Input: part model. Units: mm. Frame: model coordinates. A direction names the side the tool comes from. Round coordinates to 2 decimals unless told otherwise and drop trailing zeros. Loops run counter-clockwise (first coordinate to the right, second up) from the corner with the lowest first, then second, coordinate; pieces in that order, holes last.
1) Draft query along X for faces 1 (the face through (-53, 1, 35.19)), 2 (the face through (46.445, 1.479, 54.256)), 3 (the face through (42, 1, 38.19)). Return one class per face: pulls with the +X half, pulls with the -X half, needs draft (parallel to the pull), parting line crosses it, or undercut.
2) Ray query, line 1 along X through (y, z) = (0.4, 41); line 2 along X through (y, z) = (2.6, 54); line 3 along X through (y, z) = (1.25, 37.5). Return the intervals inside material, ascending.
3) Section A-A, the plane z = 45.5. Return loops of the section in (x, y).
4) Section D-D, the plane x = 26. Return loops of the section in (y, z).
5) First-contact query: pin 1 (0.9 mm diameter, centred on x = -47, y = 2, fed in from -Z); pin 2 (1.5 mm diameter, centred on x = 3.5, y = 2, fed in from -Z); pin 3 (0.9 mm diameter, centred on y = 1.5, z = 41.5, fed in from +X); pin 4 (0.9 mm diameter, centred on y = 1.5, z = 47, fed in from +X). Flat tips, straight axial feed; report the tip coordinate or a pass-through.
6) Section B-B, the plane y = 1.2. State how many separate pieces and enclosed holes the cut face has, and give its area (3 significant figures).
7) Access query for faces 4 (the face through (-55.419, 1, 41)), 5 (the face through (18.229, 1.521, 62.266)), 6 (the face through (31.581, 1, 58)). Directions: +Z, -Z, +X, -X, +Y, -Y. A direction counts if a zero-diameter tool reaches every point of the face in a straight line with its end or side. Return the directions, or none.
8) Section C-C, the plane x = 6. Return loops of the section in (y, z).
from build123d import *

# Parameters (mm, degrees)
BOSS_EXTRUDE1_DEPTH = 3
FILLET2_R           = 2.5
FILLET3_R           = 1
FILLET5_R           = 2.5
FILLET6_R           = 5
FILLET7_R           = 25


with BuildPart() as part:
    # Sketch1 → Boss-Extrude1 (new body)
    with BuildSketch(Plane(origin=(0, 0, 0), x_dir=(1, 0, 0), z_dir=(0, 1, 0))):
        with BuildLine():
            Line((-62.418566214, -47.190177149), (-58.418566214, -47.190177149))
            Line((-58.418566214, -47.190177149), (-58.418566214, -35.190177149))
            Line((-58.418566214, -35.190177149), (-48.418566214, -35.190177149))
            Line((-48.418566214, -35.190177149), (-48.418566214, -47.190177149))
            Line((-48.418566214, -47.190177149), (-44.418566214, -47.190177149))
            Line((-44.418566214, -47.190177149), (-43.418817081, -57.187668474))
            Line((-43.418817081, -57.187668474), (-43.418817081, -59.137504987))
            Line((-43.418817081, -59.137504987), (-40.418817081, -59.137504987))
            Line((-40.418817081, -59.137504987), (-40.418817081, -57.137504987))
            Line((-40.418817081, -57.137504987), (-38.722684913, -52.023499684))
            ThreePointArc((-38.722684913, -52.023499684), (-37.561438496, -51.091888176), (-36.235977812, -51.769787298))
            Line((-36.235977812, -51.769787298), (-33.13692456, -57.137504987))
            Line((-33.13692456, -57.137504987), (28.581433786, -57.137504987))
            Line((28.581433786, -57.137504987), (28.581433786, -59.137504987))
            Line((28.581433786, -59.137504987), (31.581433786, -59.137504987))
            Line((31.581433786, -59.137504987), (31.581433786, -57.187643384))
            Line((31.581433786, -57.187643384), (32.581433786, -47.190177149))
            Line((32.581433786, -47.190177149), (36.581433786, -47.190177149))
            Line((36.581433786, -47.190177149), (36.581433786, -35.190177149))
            Line((36.581433786, -35.190177149), (46.581433786, -35.190177149))
            Line((46.581433786, -35.190177149), (46.581433786, -47.190177149))
            Line((46.581433786, -47.190177149), (50.581433786, -47.190177149))
            Line((50.581433786, -47.190177149), (41.830568429, -62.137504987))
            ThreePointArc((41.830568429, -62.137504987), (30.081433786, -65.137504987), (18.332299143, -62.137504987))
            Line((18.332299143, -62.137504987), (-26.340663857, -62.360316421))
            ThreePointArc((-26.340663857, -62.360316421), (-40.074739293, -66.344446247), (-53.758312176, -62.190177149))
            Line((-53.758312176, -62.190177149), (-62.202371167, -57.642224353))
            ThreePointArc((-62.202371167, -57.642224353), (-62.450096964, -57.079754395), (-61.965274707, -56.702013871))
            Line((-61.965274707, -56.702013871), (-59.524980934, -56.702013871))
            ThreePointArc((-59.524980934, -56.702013871), (-58.225942828, -55.952013871), (-58.225942828, -54.452013871))
            Line((-58.225942828, -54.452013871), (-62.418566214, -47.190177149))
        make_face()
        Polygon((36.547763078, -51.190177149), (39.581433786, -51.190177149), (39.581433786, -44.190177149), (39.581433786, -38.190177149), (43.581433786, -38.190177149), (43.581433786, -44.229690019), (43.581433786, -51.229690019), (40.093369012, -57.187643384), (35.947864455, -57.187643384), align=None, mode=Mode.SUBTRACT)
        Polygon((-55.418566214, -38.190177149), (-51.418566214, -38.190177149), (-51.418566214, -44.190177149), (-51.418566214, -51.190177149), (-48.038516462, -51.190177149), (-47.438516462, -57.190177149), (-52.026261368, -57.190177149), (-55.490362984, -51.190177149), (-55.418566214, -44.190545357), align=None, mode=Mode.SUBTRACT)
    extrude(amount=BOSS_EXTRUDE1_DEPTH)

    # Fillet2
    fillet2_edges = [part.edges().sort_by_distance(p)[0] for p in [
        (-58.418566214, 1.5, 35.190177149),
        (-48.418566214, 1.5, 35.190177149),
        (36.581433786, 1.5, 35.190177149),
        (46.581433786, 1.5, 35.190177149),
    ]]
    fillet(fillet2_edges, radius=FILLET2_R)

    # Fillet3
    fillet3_edges = [part.edges().sort_by_distance(p)[0] for p in [
        (-33.13692456, 1.5, 57.137504987),
    ]]
    fillet(fillet3_edges, radius=FILLET3_R)

    # Fillet5
    # the kernel refuses this fillet: 2.5 mm, written as the material it adds along each edge
    with BuildSketch(Plane(origin=(-53.758312176, 0, 62.190177149), x_dir=(0.835787745770118, 0, 0.5490526787299234), z_dir=(0, 1, 0))) as fillet5_piece_1:
        with BuildLine():
            CenterArc((0.109109334, -2.499994653), FILLET5_R, 90.11850268, 4.876730224)
            Line((-0.10857281, -0.009489788), (0, 0))
            ThreePointArc((0, 0), (0.051969341, -5.3743e-05), (0.103938683, 0))
        make_face()
    extrude(amount=3)
    # the kernel refuses this fillet: 2.5 mm, written as the material it takes off along each edge
    with BuildSketch(Plane(origin=(41.830568429, -1.88265381, 62.137504987), x_dir=(0.5052312330715905, 0, -0.8629840097759403), z_dir=(0, 1, 0))) as fillet5_2_piece_1:
        with BuildLine():
            CenterArc((0.713618061, 2.5), FILLET5_R, 237.2334899, 32.7665101)
            ThreePointArc((-0.639423937, 0.397792267), (-0.321239998, 0.19643993), (0, 0))
            Line((0, 0), (0.713618061, 0))
        make_face()
    extrude(amount=6.76530762, mode=Mode.SUBTRACT)

    # Fillet6
    fillet6_edges = [part.edges().sort_by_distance(p)[0] for p in [
        (18.332299143, 1.5, 62.137504987),
    ]]
    fillet(fillet6_edges, radius=FILLET6_R)

    # Fillet7
    fillet7_edges = [part.edges().sort_by_distance(p)[0] for p in [
        (-26.340663857, 1.5, 62.360316421),
    ]]
    fillet(fillet7_edges, radius=FILLET7_R)


solid = part.part
Final values:
1. face 1: needs draft
1. face 2: pulls with the +X half
1. face 3: undercut
2. line 1: x = -58.42 to -55.42, -51.42 to -48.42, 36.58 to 39.58, 43.58 to 46.58
2. line 2: x = -58.49 to -53.87, -47.76 to -43.74, -39.38 to -34.95, 31.9 to 36.27, 41.96 to 46.59
2. line 3: x = -58.41 to -48.43, 36.59 to 46.57
3. outline: (-58.42, 0) - (-55.43, 0) - (-55.43, 3) - (-58.42, 3) - close; (-51.42, 0) - (-48.42, 0) - (-48.42, 3) - (-51.42, 3) - close; (36.58, 0) - (39.58, 0) - (39.58, 3) - (36.58, 3) - close; (43.58, 0) - (46.58, 0) - (46.58, 3) - (43.58, 3) - close
4. outline: (0, 57.14) - (3, 57.14) - (3, 64.8) - (0, 64.8) - close
5. pin 1: stops at z = 47.19
5. pin 2: stops at z = 57.14
5. pin 3: stops at x = 46.58
5. pin 4: stops at x = 50.58
6. separate pieces: 1
6. enclosed holes: 2
6. area: 1,030 mm2
7. face 4: +Y, -Y
7. face 5: +Z, +Y, -Y
7. face 6: -Z, +Y, -Y
8. outline: (0, 57.14) - (3, 57.14) - (3, 62.2) - (0, 62.2) - close
